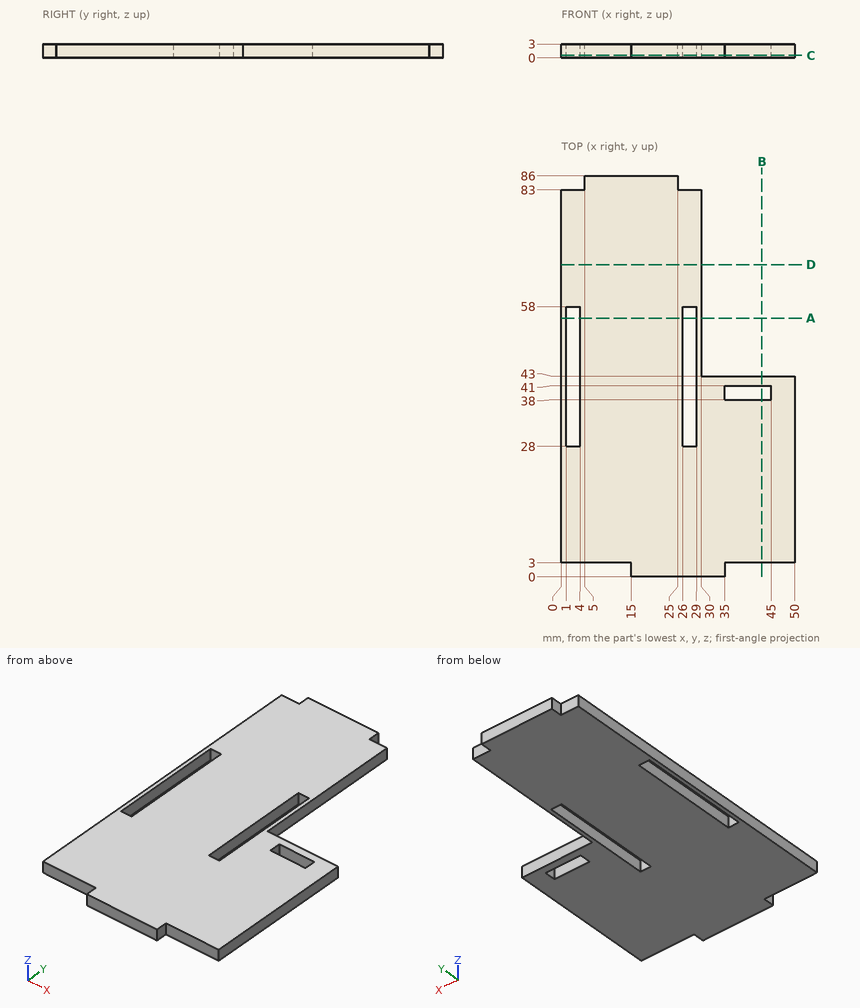
Geometry check sheet. Reference: drawing and pictorial views, mm from the part's lowest x, y, z. Round coordinates to 2 decimals unless told otherwise and drop trailing zeros. Order: outer loops, then holes, each group sorted by start corner. A loop starts at its lowest first (then second) coordinate and runs counter-clockwise, first axis right, second up. Notation, with made-up numbers: (-36.5, 54) - (-0.5, 54) arc R36 ccw to (-0.5, 90) - close; hole circle Ø8 at (-24, -25). An arc over 180 degrees is marked (long way). One line per question, with ' | ' between items. Start each with the question number.
(1) Sectioned sample at D-D on y = 67. Record the cut outline in (x, z), and give its area (3 significant figures).
(2) Sectioned sample at B-B on x = 43. Record the cut outline in (y, z).
(3) Sectioned sample at C-C on z = 0.55. Record the cut outline in (x, y), and give its area (3 significant figures).
(4) Thickness scan on L1, parallel to X at y = 46, z = 2.5; L2, parallel to X at y = 37, z = 0.4; L3, parallel to Y at x = 28, z = 2.6. Record the ranges inside material, lowest first. Write a range as [from, to].
(5) Depth check by flat-ended pin: pin 1 Ø1.5 at (y, z) = (1, 1) entering from +X; pin 2 Ø1.5 at (y, z) = (52.5, 0.5) entering from +X; pin 3 Ø0.9 at (x, z) = (41.5, 2) entering from +Y. Enter the tip coordinate at first touch or a pass-through.
(6) Sectioned sample at A-A on y = 55.5. Record the cut outline in (x, z).
Conclusion:
1) outline: (0, 0) - (30, 0) - (30, 3) - (0, 3) - close | area: 90.0 mm2
2) outline: (3, 0) - (38, 0) - (38, 3) - (3, 3) - close; (41, 0) - (43, 0) - (43, 3) - (41, 3) - close
3) outline: (0, 3) - (15, 3) - (15, 0) - (35, 0) - (35, 3) - (50, 3) - (50, 43) - (30, 43) - (30, 83) - (25, 83) - (25, 86) - (5, 86) - (5, 83) - (0, 83) - close; hole (1, 28) - (4, 28) - (4, 58) - (1, 58) - close; hole (26, 28) - (29, 28) - (29, 58) - (26, 58) - close; hole (35, 38) - (45, 38) - (45, 41) - (35, 41) - close | area: 3,110 mm2
4) L1: x = [0, 1], [4, 26], [29, 30] | L2: x = [0, 1], [4, 26], [29, 50] | L3: y = [0, 28], [58, 83]
5) pin 1: stops at x = 35 | pin 2: stops at x = 30 | pin 3: stops at y = 43
6) outline: (0, 0) - (1, 0) - (1, 3) - (0, 3) - close; (4, 0) - (26, 0) - (26, 3) - (4, 3) - close; (29, 0) - (30, 0) - (30, 3) - (29, 3) - close
